from build123d import *

# Parameters (mm, degrees)
F0_R     = 7.6
F1_DEPTH = 25
F2_R     = 1.5
F3_DEPTH = 44.701
F4_R     = 5


with BuildPart() as f1:
    # F0 (on Top) → F1 (new body)
    with BuildSketch(Plane.XY):
        with BuildLine():
            ThreePointArc((-84.206832, -4), (-69.75, -15), (-55.293168, -4))
            Line((-55.293168, -4), (55.293168, -4))
            ThreePointArc((55.293168, -4), (69.75, -15), (84.206832, -4))
            Line((84.206832, -4), (92, -4))
            Line((92, -4), (92, 29.7))
            Line((92, 29.7), (-92, 29.7))
            Line((-92, 29.7), (-92, -4))
            Line((-92, -4), (-84.206832, -4))
        make_face()
        with Locations((-69.75, 0)):
            Circle(F0_R, mode=Mode.SUBTRACT)
        with Locations((69.75, 0)):
            Circle(F0_R, mode=Mode.SUBTRACT)
    extrude(amount=F1_DEPTH)

    # F2 (on face) → F3 (cut, through all)
    with BuildSketch(Plane(origin=(0, 29.7, 0), x_dir=(-1, 0, 0), z_dir=(0, 1, 0))):
        with Locations((55, 12.5)):
            Circle(F2_R)
        with Locations((-55, 12.5)):
            Circle(F2_R)
        with Locations((85, 12.5)):
            Circle(F2_R)
        with Locations((-85, 12.5)):
            Circle(F2_R)
    extrude(amount=-F3_DEPTH, mode=Mode.SUBTRACT)

    # F4
    f4_edges = [f1.edges().sort_by_distance(p)[0] for p in [
        (-92, -4, 12.5),
        (92, -4, 12.5),
    ]]
    fillet(f4_edges, radius=F4_R)


solid = f1.part
Input: part model. Units: mm. Frame: model coordinates. A direction names the side the tool comes from. Give positions to 0.01 mm unless a question says otherwise; leave off trailing zeros. Loops run counter-clockwise (first coordinate to the right, second up) from the corner with the lowest first, then second, coordinate; pieces in that order, holes last. Notation, with made-up numbers: M 40.25,72.5 L 62.25,72.5 A23 cw 62.25,96.5 Z; hole C 45.25,-15.75 d6. An arc over 180 degrees is marked long. Use one line per item in the form item = value.
1. Section query B-B, the plane z = 9. Return the cut outline in (x, y).
Numbers:
outline = M -92,1 A5 ccw -87,-4 L -84.21,-4 A15 ccw -55.29,-4 L 55.29,-4 A15 ccw 84.21,-4 L 87,-4 A5 ccw 92,1 L 92,29.7 L -92,29.7 Z; hole C -69.75,0 d15.2; hole C 69.75,0 d15.2
2. Line query: L1, parallel to Z at x = 85, y = 17.5; L2, parallel to Y at x = 69.75, z = 19.5; L3, parallel to X at y = -7, z = 10.5. Output: solid intervals per line, ascending.
Numbers:
L1 = 0 to 11, 14 to 25
L2 = -15 to -7.6, 7.6 to 29.7
L3 = -83.02 to -72.71, -66.79 to -56.48, 56.48 to 66.79, 72.71 to 83.02
3. Section query C-C, the plane y = 5.5. Return the cut outline in (x, z) (3 decimals).
Numbers:
outline = M -92,0 L -74.995,0 L -74.995,25 L -92,25 Z; M -64.505,0 L 64.505,0 L 64.505,25 L -64.505,25 Z; M 74.995,0 L 92,0 L 92,25 L 74.995,25 Z; hole C -85,12.5 d3; hole C -55,12.5 d3; hole C 55,12.5 d3; hole C 85,12.5 d3
4. Pull-direction query (Y, two-part tool) for faces 3 (the face through (-70.023, -14.998, 12.325)), 4 (the face through (-86.43, 12.1, 12.95)), 5 (the face through (-77.343, 0.334, 12.325)); classes: released by +Y, released by -Y, zero draft, split by the parting line, or undercut.
Numbers:
face_3 = released by -Y
face_4 = zero draft
face_5 = undercut
5. Section query A-A, the plane x = -69.75. Return the cut outline in (y, z), and give its area (4 significant figures).
Numbers:
outline = M -15,0 L -7.6,0 L -7.6,25 L -15,25 Z; M 7.6,0 L 29.7,0 L 29.7,25 L 7.6,25 Z
area = 737.5 mm²
6. Reachability of faces 1 (the face through (-1, 13, 0)), 2 (the face through (-1, -4, 12)) from +Z, -Z, +X, -X, +Y, -Y: full face, straight path, thin tool, end or side. Return the list, or none.
Numbers:
face_1 = -Z, +X, -X, +Y, -Y
face_2 = +Z, -Z, -Y
7. First-contact query: pin 1 (2 mm diameter, centred on x = -85.5, z = 11.5, fed in from -Y); pin 2 (5 mm diameter, centred on x = -85, z = 12.5, fed in from -Y); pin 3 (3.5 mm diameter, centred on x = 85, z = 12.5, fed in from -Y). Flat tips, straight axial feed; report the tip coordinate or a pass-through.
Numbers:
pin_1 = -4
pin_2 = -7.9
pin_3 = -6.54
